```python
from build123d import *

# Parameters (mm, degrees)
SKETCH6_R                                = 66.04
BOSS_EXTRUDE1_DEPTH                      = 2.54
PIPE_TAP_DRILL_FOR_1_4_TAP_RELIEF_VALV_D = 11.1252
PIPE_TAP_DRILL_FOR_1_4_TAP_VENT_VALVE_D  = 11.1252


with BuildPart() as part:
    # Sketch1 → Revolve1 (revolve)
    with BuildSketch(Plane.XY, mode=Mode.PRIVATE) as revolve1_sk:
        Polygon((0, 0), (72.898, 0), (72.898, 2.4638), (69.977, 2.4638), (69.977, 7.4422), (72.898, 7.4422), (72.898, 9.906), (69.977, 9.906), (69.977, 14.986), (72.898, 14.986), (72.898, 17.3482), (66.548, 17.3482), (66.548, 6.35), (0, 6.35), align=None)
    revolve(revolve1_sk.sketch.rotate(Axis((0, 48.192213231, 0), (0, -1, 0)), 180), axis=Axis((0, 48.192213231, 0), (0, -1, 0)))

    # Sketch6 → Boss-Extrude1 (add)
    with BuildSketch(Plane.XZ):
        Circle(SKETCH6_R)
    extrude(amount=BOSS_EXTRUDE1_DEPTH)

    # Pipe Tap Drill for 1/4 Tap - Relief Valve (through all)
    with Locations(Plane(origin=(0, -2.54, 0), x_dir=(-1, 0, 0), z_dir=(0, -1, 0))):
        with Locations((0, 44.958)):
            Hole(PIPE_TAP_DRILL_FOR_1_4_TAP_RELIEF_VALV_D / 2)

    # Pipe Tap Drill for 1/4 Tap - Vent Valve (through all)
    with Locations(Plane(origin=(0, -2.54, 0), x_dir=(-1, 0, 0), z_dir=(0, -1, 0))):
        with Locations((0, -44.958)):
            Hole(PIPE_TAP_DRILL_FOR_1_4_TAP_VENT_VALVE_D / 2)


solid = part.part
```
Build history of the part. All positions in model axes, mm. A direction names the side the tool comes from. Round coordinates to 2 decimals unless told otherwise and drop trailing zeros. Order: outer loops, then holes, each group sorted by start corner. A loop starts at its lowest first (then second) coordinate and runs counter-clockwise, first axis right, second up. Notation, with made-up numbers: (-36.75, 9.5) -> (-15.75, 9.5) arc R27 cw to (-15.75, 29.5) -> close; hole circle Ø10 at (-25.75, 3). An arc over 180 degrees is marked (long way). Answer in a Markdown table with one row per item.
1) Band-saw the part on A-A on z = 0. Give the cut face in (x, y), and give its area (3 significant figures).
Values:
| item | result |
|---|---|
| outline | (-72.9, 0) -> (-66.04, 0) -> (-66.04, -2.54) -> (66.04, -2.54) -> (66.04, 0) -> (72.9, 0) -> (72.9, 2.46) -> (69.98, 2.46) -> (69.98, 7.44) -> (72.9, 7.44) -> (72.9, 9.91) -> (69.98, 9.91) -> (69.98, 14.99) -> (72.9, 14.99) -> (72.9, 17.35) -> (66.55, 17.35) -> (66.55, 6.35) -> (-66.55, 6.35) -> (-66.55, 17.35) -> (-72.9, 17.35) -> (-72.9, 14.99) -> (-69.98, 14.99) -> (-69.98, 9.91) -> (-72.9, 9.91) -> (-72.9, 7.44) -> (-69.98, 7.44) -> (-69.98, 2.46) -> (-72.9, 2.46) -> close |
| area | 1,340 mm2 |
2) Band-saw the part on B-B on x = -8. Give the cut face in (y, z), and give its area (3 significant figures).
Values:
| item | result |
|---|---|
| outline | (-2.54, -65.55) -> (0, -65.55) -> (0, -72.46) -> (2.46, -72.46) -> (2.46, -69.52) -> (7.44, -69.52) -> (7.44, -72.46) -> (9.91, -72.46) -> (9.91, -69.52) -> (14.99, -69.52) -> (14.99, -72.46) -> (17.35, -72.46) -> (17.35, -66.07) -> (6.35, -66.07) -> (6.35, 66.07) -> (17.35, 66.07) -> (17.35, 72.46) -> (14.99, 72.46) -> (14.99, 69.52) -> (9.91, 69.52) -> (9.91, 72.46) -> (7.44, 72.46) -> (7.44, 69.52) -> (2.46, 69.52) -> (2.46, 72.46) -> (0, 72.46) -> (0, 65.55) -> (-2.54, 65.55) -> close |
| area | 1,330 mm2 |
3) Mould opens along Z. For faces 5 (the flat face through (-1, -2.54, 1)), 6 (the cylindrical face through (-66.746, 4.988, -21.019)), 7 (the cylindrical face through (-1.206, 1.967, 50.388)) say: released by +Z, released by -Z, zero draft, split by the parting line, or undercut.
Values:
| item | result |
|---|---|
| face 5 | zero draft |
| face 6 | split by the parting line |
| face 7 | undercut |
4) Which spindle directions (+Z, -Z, +X, -X, +Y, -Y) get a long thin tool onto all of the face, cutting with end or side? Do faces 1 (the cylindrical face through (63, -1.3, 19.8)), 2 (the cylindrical face through (15.803, 1.249, 71.165)), 3 (the cylindrical face through (-66.746, 12.482, -21.019)), 4 (the cylindrical face through (8.663, 11.772, -65.982)). Say none if no direction does.
Values:
| item | result |
|---|---|
| face 1 | -Y |
| face 2 | +Y, -Y |
| face 3 | none |
| face 4 | +Y |
5) Wall check: L1, parallel to Y at x = -34.5, z = 61.5; L2, parallel to Z at x = -0.5, y = 16.25; L3, parallel to Z at x = 0, y = 14.75. Give the ranges that are in metal, low to high.
Values:
| item | result |
|---|---|
| L1 | 0 to 2.46, 7.44 to 9.91, 14.99 to 17.35 |
| L2 | -72.9 to -66.55, 66.55 to 72.9 |
| L3 | -69.98 to -66.55, 66.55 to 69.98 |
6) Pin check, flat tips, straight feed: P1, Ø9, axis at x = 0, z = 44.958, coming from the -Y side; P2, Ø3, axis at x = 3.5, y = 6, coming from the +Z side; P3, Ø5, axis at x = -9.5, y = 13, coming from the -Z side; P4, Ø6, axis at y = 2.5, z = -40, coming from the +X side. Stop position of each tip, or through.
Values:
| item | result |
|---|---|
| P1 | through |
| P2 | z = 72.83 |
| P3 | z = -72.46 |
| P4 | x = 62.81 |
